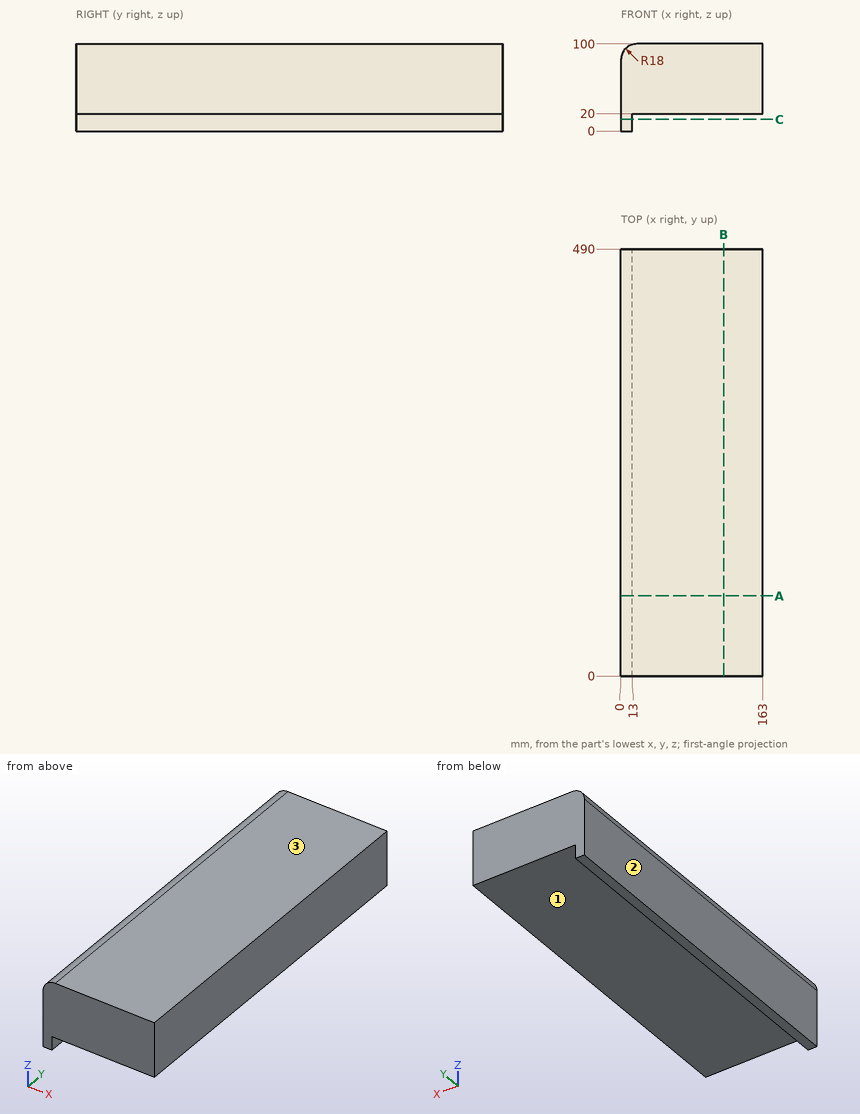
Could you check a few things on this drawing? It's one solid part, dimensions in mm from its lowest x, y, z. Round coordinates to 2 decimals unless told otherwise and drop trailing zeros. Loops run counter-clockwise (first coordinate to the right, second up) from the corner with the lowest first, then second, coordinate; pieces in that order, holes last.
Q1. I want a section at C-C (z = 13.5). Write out the boundary of the cut face in (x, y), and give its area (3 significant figures).
Q2. I want a section at A-A (y = 92). Write out the boundary of the cut face in (x, z), and give its area (3 significant figures).
Q3. For P1, Ø1.5, axis at x = 118.5, y = 303, coming from the -Z side; P2, Ø6, axis at y = 217.5, z = 11, coming from the +X side, each with a flat end and sliding along its axis, tell me the tip position at first contact or that it passes through.
Q4. Thinking about a two-plate mould opening in Z: for the marked faces 1, 2 and 3, which applies, pulls with the +Z half, pulls with the -Z half, needs draft (parallel to the pull), parting line crosses it, or undercut?
Q5. I want a section at B-B (x = 118). Write out the boundary of the cut face in (y, z).
Q6. Please list where these lines run through material, in increasing order: L1, parallel to Z at x = 110, y = 132.5; L2, parallel to X at y = 29, z = 18; L3, parallel to X at y = 84, z = 84.
Answer below:
1. outline: (0, 0) - (13, 0) - (13, 490) - (0, 490) - close
1. area: 6,370 mm2
2. outline: (0, 0) - (13, 0) - (13, 20) - (163, 20) - (163, 100) - (18, 100) arc R18 ccw to (0, 82) - close
2. area: 13,200 mm2
3. P1: stops at z = 20
3. P2: stops at x = 13
4. face 1: pulls with the -Z half
4. face 2: needs draft
4. face 3: pulls with the +Z half
5. outline: (0, 20) - (490, 20) - (490, 100) - (0, 100) - close
6. L1: z = 20 to 100
6. L2: x = 0 to 13
6. L3: x = 0.11 to 163
